Source: CAD feature listing. Evaluate the final solid. Frame: model axes, mm. A direction names the side the tool comes from. Round coordinates to 2 decimals unless told otherwise and drop trailing zeros. Order: outer loops, then holes, each group sorted by start corner. A loop starts at its lowest first (then second) coordinate and runs counter-clockwise, first axis right, second up. Notation, with made-up numbers: M 41.25,72.25 L 62.25,72.25 A23 ccw 62.25,106.25 Z; hole C 57.5,-21.75 d4. An arc over 180 degrees is marked long. Answer in a Markdown table with one row per item. Add a question column.
```python
from build123d import *

# Parameters (mm, degrees)
SKETCH1_R                  = 0.8
BRACKETWITHBOLTHOLES_DEPTH = 2.5
SKETCH2_W                  = 10
SKETCH2_H                  = 2
BRACKETEXTENSION_DEPTH     = 2.5
SKETCH2_3_W                = 10
SKETCH2_3_H                = 2
BASE_DEPTH                 = 5
BASE_DEPTH_BACK            = 7.5
SKETCH3_R                  = 1
BASEBOLTHOLES_DEPTH        = 3
SKETCH3_3_R                = 1
BASENUTSLOTS_DEPTH         = 1
SKETCH4_W                  = 1.5
SKETCH4_H                  = 10
STIFFENERRIB_DEPTH         = 42.5
BRACKETNUTSLOTS_DEPTH      = 1.5


with BuildPart() as part:
    # Sketch1 → BracketWithBoltHoles (new body)
    with BuildSketch(Plane.XY):
        Polygon((-10.5, 17.5), (-10.5, 11.5), (-3.5, 11.5), (-3.5, -11.5), (-10.5, -11.5), (-10.5, -17.5), (10.5, -17.5), (10.5, -11.5), (3.5, -11.5), (3.5, 11.5), (10.5, 11.5), (10.5, 17.5), align=None)
        with Locations((-8, -15)):
            Circle(SKETCH1_R, mode=Mode.SUBTRACT)
        with Locations((8, -15)):
            Circle(SKETCH1_R, mode=Mode.SUBTRACT)
        with Locations((-8, 15)):
            Circle(SKETCH1_R, mode=Mode.SUBTRACT)
        with Locations((8, 15)):
            Circle(SKETCH1_R, mode=Mode.SUBTRACT)
    extrude(amount=BRACKETWITHBOLTHOLES_DEPTH)

    # Sketch2 → BracketExtension (add)
    with BuildSketch(Plane.XY.offset(2.5)):
        Polygon((10.5, -17.5), (-10.5, -17.5), (-10.5, -25), (-5, -25), (-5, -23), (5, -23), (5, -25), (10.5, -25), align=None)
        with Locations((0, -24)):
            Rectangle(SKETCH2_W, SKETCH2_H)
    extrude(amount=-BRACKETEXTENSION_DEPTH)

    # Sketch2<3> → Base (add, two sides)
    with BuildSketch(Plane.XY.offset(2.5)) as base_sk:
        with Locations((0, -24)):
            Rectangle(SKETCH2_3_W, SKETCH2_3_H)
    extrude(amount=BASE_DEPTH)
    extrude(base_sk.sketch, amount=-BASE_DEPTH_BACK)

    # Sketch3 → BaseBoltHoles (cut, through all)
    with BuildSketch(Plane(origin=(0, -23, 0), x_dir=(1, 0, 0), z_dir=(0, 1, 0))):
        with Locations((0, -5)):
            Circle(SKETCH3_R)
        with Locations((0, 2.5)):
            Circle(SKETCH3_R)
    extrude(amount=-BASEBOLTHOLES_DEPTH, mode=Mode.SUBTRACT)

    # Sketch3<3> → BaseNutSlots (cut)
    with BuildSketch(Plane(origin=(0, -23, 0), x_dir=(1, 0, 0), z_dir=(0, 1, 0))):
        Polygon((1.154700538, -7), (2.309401077, -5), (1.154700538, -3), (-1.154700538, -3), (-2.309401077, -5), (-1.154700538, -7), align=None)
        with Locations((0, -5)):
            Circle(SKETCH3_3_R, mode=Mode.SUBTRACT)
        Polygon((-1.154700538, 0.5), (-2.309401077, 2.5), (-1.154700538, 4.5), (1.154700538, 4.5), (2.309401077, 2.5), (1.154700538, 0.5), align=None)
        with Locations((0, 2.5)):
            Circle(SKETCH3_3_R, mode=Mode.SUBTRACT)
    extrude(amount=-BASENUTSLOTS_DEPTH, mode=Mode.SUBTRACT)

    # Sketch4 → StiffenerRib (add)
    with BuildSketch(Plane(origin=(0, 17.5, 0), x_dir=(1, 0, 0), z_dir=(0, 1, 0))):
        with Locations((-11.25, -1.25)):
            Rectangle(SKETCH4_W, SKETCH4_H)
    stiffenerrib = extrude(amount=-STIFFENERRIB_DEPTH)

    # StiffenerRib2: StiffenerRib across plane
    add(stiffenerrib.mirror(Plane(origin=(0, 0, 0), x_dir=(0, 0, 1), z_dir=(1, 0, 0))))

    # Sketch5 → BracketNutSlots (cut)
    with BuildSketch(Plane.XY.offset(2.5)):
        Polygon((-7.278312164, 16.25), (-8.721687836, 16.25), (-9.443375673, 15), (-8.721687836, 13.75), (-7.278312164, 13.75), (-6.556624327, 15), align=None)
        Polygon((-7.278312164, -13.75), (-8.721687836, -13.75), (-9.443375673, -15), (-8.721687836, -16.25), (-7.278312164, -16.25), (-6.556624327, -15), align=None)
        Polygon((8.721687836, -16.25), (7.278312164, -16.25), (6.556624327, -15), (7.278312164, -13.75), (8.721687836, -13.75), (9.443375673, -15), align=None)
        Polygon((6.556624327, 15), (7.278312164, 16.25), (8.721687836, 16.25), (9.443375673, 15), (8.721687836, 13.75), (7.278312164, 13.75), align=None)
    extrude(amount=-BRACKETNUTSLOTS_DEPTH, mode=Mode.SUBTRACT)


solid = part.part
```
(1) Cut plane A-A (y = 8.5). Return loops of the section in (x, z), and give its area (3 significant figures).
(2) Pin query (flat end, axial travel): pin 1 (5 mm diameter, centred on x = -9, z = -1.5, fed in from +Y); pin 2 (1.3 mm diameter, centred on x = -8, y = -15, fed in from -Z); pin 3 (4 mm diameter, centred on x = 5, y = 4.5, fed in from -Z); pin 4 (1.2 mm diameter, centred on x = -0.5, z = 4.5, fed in from +Y). Return the tip coordinate at first contact, or that it passes through.
(3) Cut plane C-C (z = 1.5). Count the separate pieces of the cut face and the enclosed holes in it, and give its area (3 significant figures).
(4) Cut plane B-B (x = 0). Return loops of the section in (y, z), and give its area (3 significant figures).
(5) Line query: line 1 (Y direction, x = 8, z = 0.7); line 2 (X direction, y = -15, z = 0.4); line 3 (X direction, y = -24.35, z = -2.5). Output: solid intervals per line, ascending. Write a range as from..to.
(6) Draft query along Z for faces 1 (the face through (0, -23.5, -0.5)), 2 (the face through (-0.13, -24.49, 4.01)), 3 (the face through (9.08, -14.37, 1.76)), 4 (the face through (-11, -3, -3.75)). Return one class per face: +Z half, -Z half, draft (parallel to the pull), parting line (faces both ways), or undercut.
(7) Access query for faces 5 (the face through (7, 11.5, 1)), 6 (the face through (-6.912, -14.384, 1.76)), 7 (the face through (1.74, -23.49, 4.01)). Directions: +Z, -Z, +X, -X, +Y, -Y. A direction counts if a zero-diameter tool reaches every point of the face in a straight line with its end or side. Return the directions, or none.
Answer list:
| question | item | result |
|---|---|---|
| 1 | outline | M -12,-3.75 L -10.5,-3.75 L -10.5,6.25 L -12,6.25 Z; M -3.5,0 L 3.5,0 L 3.5,2.5 L -3.5,2.5 Z; M 10.5,-3.75 L 12,-3.75 L 12,6.25 L 10.5,6.25 Z |
| 1 | area | 47.5 mm² |
| 2 | pin 1 | y = 17.5 |
| 2 | pin 2 | through |
| 2 | pin 3 | z = 0 |
| 2 | pin 4 | y = -24 |
| 3 | separate pieces | 1 |
| 3 | enclosed holes | 6 |
| 3 | area | 676 mm² |
| 4 | outline | M -25,-5 L -23,-5 L -23,-4.5 L -24,-4.5 L -24,-3.5 L -25,-3.5 Z; M -25,-1.5 L -24,-1.5 L -24,-0.5 L -23,-0.5 L -23,0 L 17.5,0 L 17.5,2.5 L -23,2.5 L -23,3 L -24,3 L -24,4 L -25,4 Z; M -25,6 L -24,6 L -24,7 L -23,7 L -23,7.5 L -25,7.5 Z |
| 4 | area | 114 mm² |
| 5 | line 1 | -25..-15.8, -14.2..-11.5, 11.5..14.2, 15.8..17.5 |
| 5 | line 2 | -12..-8.8, -7.2..7.2, 8.8..12 |
| 5 | line 3 | -12..-10.5, -5..-1, 1..5, 10.5..12 |
| 6 | face 1 | undercut |
| 6 | face 2 | undercut |
| 6 | face 3 | draft |
| 6 | face 4 | -Z half |
| 7 | face 5 | +Z, -Z |
| 7 | face 6 | +Z |
| 7 | face 7 | +Y |
